Work out the finished part from the listing and answer in its coordinate system (mm). A direction names the side the tool comes from. Coordinates: 2 decimals unless noted, no trailing zeros. Order: outer loops, then holes, each group sorted by start corner. A loop starts at its lowest first (then second) coordinate and runs counter-clockwise, first axis right, second up. Notation, with made-up numbers: (12, 13) -> (34, 13) arc R22 ccw to (34, 40) -> close; hole circle Ø1 at (-25.75, -6). An arc over 180 degrees is marked (long way). Write item = value, one per line. Start each with the question number.
Q1. The part is cut by section A-A, the plane y = 0. Determine the outline of the cut face in (x, z), plus the area to 3 significant figures.
Q2. The part is cut by section B-B, the plane x = 0. Determine the outline of the cut face in (y, z).
Q3. Straight lines are drawn through the part: L1, parallel to Z at x = 0, y = 1; L2, parallel to X at y = 2.5, z = 35.2; L3, parallel to Z at x = -2.5, y = -3.5. For each, find the intervals that lie inside material, in ascending order. Write a range as from..to.
Q4. Flat-ended cylindrical pins translate along their axes: pin 1 (1.5 mm diameter, centred on x = 3, z = 35.5, fed in from +Y); pin 2 (2 mm diameter, centred on x = 4, z = 27, fed in from +Y); pin 3 (5 mm diameter, centred on y = -2.5, z = 25, fed in from +X). Find the tip coordinate at first contact, or state that the pin passes through.
Q5. The part is cut by section D-D, the plane x = -3.5. Determine the outline of the cut face in (y, z), plus the area to 3 significant figures.
Q6. Which of the six approach directions +Z, -Z, +X, -X, +Y, -Y give full straight-line access (tool end or side, diameter ignored) to faces 1 (the flat face through (-1, -3, 41.8)), 2 (the cylindrical face through (3, 0, 2)), 3 (the cylindrical face through (1.08, -4.88, 10.55))?
Q7. For a pull along Z with two mould halves and no side action, classify faces 4 (the flat face through (0, 0, 45.4)), 5 (the cylindrical face through (0.07, -0.06, 33.6)), 6 (the flat face through (0.1, -3.3, 3.6)) as +Z half, -Z half, draft (parallel to the pull), parting line (faces both ways), or undercut.
Q8. The part is cut by section C-C, the plane z = 20. Determine the outline of the cut face in (x, y).
```python
from build123d import *

# Parameters (mm, degrees)
SKETCH_1_R               = 4
EXTRUDE_1_DEPTH          = 45.4
SKETCH_2_R               = 4
SKETCH_2_R_2             = 3
CUT_EXTRUDE_1_DEPTH      = 3.6
CUT_EXTRUDE_START        = -3.6
SKETCH_3_R               = 4
SKETCH_3_R_2             = 3
CUT_EXTRUDE_2_DEPTH      = 3.6
CUT_EXTRUDE_3_DEPTH      = 46.751065561
CUT_EXTRUDE_3_DEPTH_BACK = 46.751065561
SKETCH_4_R               = 1.6
SKETCH_5_R               = 5
SKETCH_5_R_2             = 4
EXTRUDE_2_DEPTH          = 14.1


with BuildPart() as part:
    # ｽｹｯﾁ1 → ﾎﾞｽ - 押し出し1 (new body)
    with BuildSketch(Plane.XY):
        Circle(SKETCH_1_R)
    extrude(amount=EXTRUDE_1_DEPTH)

    # ｽｹｯﾁ2 → ｶｯﾄ - 押し出し1 (cut)
    with BuildSketch(Plane(origin=(0, 0, 0), x_dir=(-1, 0, 0), z_dir=(0, 0, -1))):
        Circle(SKETCH_2_R)
        Circle(SKETCH_2_R_2, mode=Mode.SUBTRACT)
    extrude(amount=-CUT_EXTRUDE_1_DEPTH, mode=Mode.SUBTRACT)

    # ｽｹｯﾁ3 → ｶｯﾄ - 押し出し2 (cut)
    with BuildSketch(Plane.XY.offset(45.4).offset(CUT_EXTRUDE_START)):
        with Locations(Location((0, 0, 0), (0, 0, 180))):
            Circle(SKETCH_3_R)
        with Locations(Location((0, 0, 0), (0, 0, 180))):
            Circle(SKETCH_3_R_2, mode=Mode.SUBTRACT)
    extrude(amount=CUT_EXTRUDE_2_DEPTH, mode=Mode.SUBTRACT)

    # ｽｹｯﾁ4 → ｶｯﾄ - 押し出し3 (cut, two sides: drawn at the far end of the back side and taken through both)
    with BuildSketch(Plane(origin=(0, 0, 0), x_dir=(1, 0, 0), z_dir=(0, 1, 0)).offset(-CUT_EXTRUDE_3_DEPTH_BACK)):
        with Locations(Location((0, -35.2, 0), (0, 0, 270))):
            Circle(SKETCH_4_R)
    extrude(amount=CUT_EXTRUDE_3_DEPTH + CUT_EXTRUDE_3_DEPTH_BACK, mode=Mode.SUBTRACT)

    # ｽｹｯﾁ5 → ﾎﾞｽ - 押し出し2 (add)
    with BuildSketch(Plane(origin=(0, 0, 3.6), x_dir=(-1, 0, 0), z_dir=(0, 0, -1))):
        Circle(SKETCH_5_R)
        Circle(SKETCH_5_R_2, mode=Mode.SUBTRACT)
    extrude(amount=-EXTRUDE_2_DEPTH)


solid = part.part
```
Model answer:
q1.outline = (-5, 3.6) -> (-3, 3.6) -> (-3, 0) -> (3, 0) -> (3, 3.6) -> (5, 3.6) -> (5, 17.7) -> (4, 17.7) -> (4, 41.8) -> (3, 41.8) -> (3, 45.4) -> (-3, 45.4) -> (-3, 41.8) -> (-4, 41.8) -> (-4, 17.7) -> (-5, 17.7) -> close; hole circle Ø3.2 at (0, 35.2)
q1.area = 369 mm2
q2.outline = (-5, 3.6) -> (-3, 3.6) -> (-3, 0) -> (3, 0) -> (3, 3.6) -> (5, 3.6) -> (5, 17.7) -> (4, 17.7) -> (4, 33.6) -> (-4, 33.6) -> (-4, 17.7) -> (-5, 17.7) -> close; (-4, 36.8) -> (4, 36.8) -> (4, 41.8) -> (3, 41.8) -> (3, 45.4) -> (-3, 45.4) -> (-3, 41.8) -> (-4, 41.8) -> close
q3.L1 = 0..33.6, 36.8..45.4
q3.L2 = -3.12..-1.6, 1.6..3.12
q3.L3 = 3.6..17.7
q4.pin_1 = 3.31
q4.pin_2 = 2.65
q4.pin_3 = 4
q5.outline = (-3.57, 3.6) -> (3.57, 3.6) -> (3.57, 17.7) -> (1.94, 17.7) -> (1.94, 41.8) -> (-1.94, 41.8) -> (-1.94, 17.7) -> (-3.57, 17.7) -> close
q5.area = 194 mm2
q6.face_1 = +Z
q6.face_2 = -Z
q6.face_3 = +Z, -Z
q7.face_4 = +Z half
q7.face_5 = undercut
q7.face_6 = -Z half
q8.outline = circle Ø8 at (0, 0)
